```python
from build123d import *

# Parameters (mm, degrees)
F0_R     = 72.5
F0_R_2   = 70.5
F1_DEPTH = 64
F0_R_3   = 68.5
F2_DEPTH = 61
F3_DEPTH = 3
F5_DEPTH = 23
F7_R     = 6.5
F8_DEPTH = 25


with BuildPart() as f1:
    # F0 (on Top) → F1 (new body)
    with BuildSketch(Plane.XY):
        Circle(F0_R)
        Circle(F0_R_2, mode=Mode.SUBTRACT)
    extrude(amount=F1_DEPTH)

    # F0 (on Top) → F2 (join)
    with BuildSketch(Plane.XY):
        Circle(F0_R_2)
        Circle(F0_R_3, mode=Mode.SUBTRACT)
    extrude(amount=F2_DEPTH)

    # F0 (on Top) → F3 (join)
    with BuildSketch(Plane.XY):
        Circle(F0_R_3)
    extrude(amount=F3_DEPTH)

    # F4 (on face) → F5 (join)
    with BuildSketch(Plane.XY.offset(3)):
        with BuildLine():
            ThreePointArc((-4.1411047216, -8.4548132206), (-9.7401828641, 19.6936534447), (16, 7))
            ThreePointArc((16, 7), (12.6936534447, -2.7401828641), (4.1411047216, -8.4548132206))
            Line((4.1411047216, -8.4548132206), (4.6587428118, -10.3866648732))
            ThreePointArc((4.6587428118, -10.3866648732), (14.2803601252, -3.9577057222), (18, 7))
            ThreePointArc((18, 7), (-10.9577057222, 21.2803601252), (-4.6587428118, -10.3866648732))
            Line((-4.6587428118, -10.3866648732), (-4.1411047216, -8.4548132206))
        make_face()
    extrude(amount=F5_DEPTH)

    # F7 (on offset) → F8 (cut)
    with BuildSketch(Plane.XZ.offset(80)):
        with Locations((0, 13)):
            Circle(F7_R)
    extrude(amount=-F8_DEPTH, mode=Mode.SUBTRACT)


solid = f1.part
```
CAD build for the part. Positions are in the model's coordinates, mm. A direction names the side the tool comes from. Round coordinates to 2 decimals unless told otherwise and drop trailing zeros. Order: outer loops, then holes, each group sorted by start corner. A loop starts at its lowest first (then second) coordinate and runs counter-clockwise, first axis right, second up. Notation, with made-up numbers: (74.5, 3) - (89.5, 3) arc R30 ccw to (89.5, 31) - close; hole circle Ø11 at (68.5, 12). An arc over 180 degrees is marked (long way). Answer in a Markdown table with one row per item. Add a question column.
(1) Band-saw the part on D-D on x = 29.5. List the corners of the cut face in (y, z), and give its area (3 significant figures).
(2) Probe L1, parallel to Z at x = 0, y = -69.5; L2, parallel to Y at x = 0, z = 61.7; L3, parallel to X at y = 7, z = 8. List the from-to ranges inside material, lowest first. Write a range as [from, to].
(3) 3-axis set-ups, long thin cutter, end or side, ignore diameter. For faces 1 (the face through (-1, 1, 0)), 2 (the face through (-6.494, -70.378, 13.286)), 3 (the face through (65.337, 20.576, 31.594)): which of +Z, -Z, +X, -X, +Y, -Y reach the whole face in a straight line?
(4) Mould opens along X. For faces 4 (the face through (69.15, 21.78, 31.55)), 5 (the face through (16, -69, 64)), 6 (the face through (-55.946, -42.898, 62.479)) say: +X half, -X half, draft (parallel to the pull), parting line (faces both ways), or undercut.
(5) Band-saw the part on B-B on z = 16.5. List the corners of the cut face in (x, y), and give its area (3 significant figures).
(6) Band-saw the part on A-A on x = 0. List the corners of the cut face in (y, z).
(7) Drop flat-ended pins along their axis: pin 1 Ø12 at (x, z) = (54, 44.5) entering from +Y; pin 2 Ø4 at (x, y) = (2, -10.5) entering from +Z; pin 3 Ø5 at (x, z) = (29.5, 19) entering from -Y. Give the stop position or say it passes through.
(8) Band-saw the part on C-C on y = 28.5. List the corners of the cut face in (x, z).
Data:
| question | item | result |
|---|---|---|
| 1 | outline | (-66.23, 0) - (66.23, 0) - (66.23, 64) - (64.03, 64) - (64.03, 61) - (61.82, 61) - (61.82, 3) - (-61.82, 3) - (-61.82, 61) - (-64.03, 61) - (-64.03, 64) - (-66.23, 64) - close |
| 1 | area | 921 mm^2 |
| 2 | L1 | z = [0, 6.5], [19.5, 61] |
| 2 | L2 | y = [-72.5, -70.5], [70.5, 72.5] |
| 2 | L3 | x = [-72.16, -68.14], [-18, -16], [16, 18], [68.14, 72.16] |
| 3 | face 1 | -Z, +X, -X, +Y, -Y |
| 3 | face 2 | -Y |
| 3 | face 3 | +Z |
| 4 | face 4 | parting line |
| 4 | face 5 | draft |
| 4 | face 6 | undercut |
| 5 | outline | (-5.48, -72.29) - (-5.48, -68.28) arc R68.5 cw (long way) to (5.48, -68.28) - (5.48, -72.29) arc R72.5 ccw (long way) to start; (-4.66, -10.39) - (-4.14, -8.45) arc R16 cw (long way) to (4.14, -8.45) - (4.66, -10.39) arc R18 ccw (long way) to start |
| 5 | area | 1,920 mm^2 |
| 6 | outline | (-72.5, 0) - (72.5, 0) - (72.5, 64) - (70.5, 64) - (70.5, 61) - (68.5, 61) - (68.5, 3) - (25, 3) - (25, 26) - (23, 26) - (23, 3) - (-68.5, 3) - (-68.5, 6.5) - (-72.5, 6.5) - close; (-72.5, 19.5) - (-68.5, 19.5) - (-68.5, 61) - (-70.5, 61) - (-70.5, 64) - (-72.5, 64) - close |
| 7 | pin 1 | stops at y = 54.33 |
| 7 | pin 2 | stops at z = 3 |
| 7 | pin 3 | stops at y = -67.28 |
| 8 | outline | (-66.66, 0) - (66.66, 0) - (66.66, 64) - (64.48, 64) - (64.48, 61) - (62.29, 61) - (62.29, 3) - (-62.29, 3) - (-62.29, 61) - (-64.48, 61) - (-64.48, 64) - (-66.66, 64) - close |
